Build history of the part. All positions in model axes, mm. Coordinates: 2 decimals unless noted, no trailing zeros. Write each loop counter-clockwise with the first axis right and the second up, starting at its lowest first coordinate (ties: lowest second). Pieces come first, ordered by that corner, then holes.
Autodesk Inventor part; units mm, degrees
ref_plane "YZ Plane" through (0, 0, 0) normal (1, 0, 0) x (0, 1, 0)
ref_plane "XZ Plane" through (0, 0, 0) normal (0, 1, 0) x (-1, 0, 0)
ref_plane "XY Plane" through (0, 0, 0) normal (0, 0, 1) x (1, 0, 0)
sketch "Sketch1" plane through (0, 0, 0) normal (1, 0, 0) x (0, 1, 0)
  circle A0 centre (0, 0) radius 57.15
  line L0 (5.3769, 1.4637) -> (3.9561, -3.9247)
  line L1 (3.9561, -3.9247) -> (-1.4208, -5.3884)
  line L2 (-1.4208, -5.3884) -> (-5.3769, -1.4637)
  line L3 (-5.3769, -1.4637) -> (-3.9561, 3.9247)
  line L4 (-3.9561, 3.9247) -> (1.4208, 5.3884)
  line L5 (1.4208, 5.3884) -> (5.3769, 1.4637)
  dimension "d0" = 114.3
  dimension "d1" = 9.652
extrude "Extrusion1" add sketch "Sketch1" along normal blind 6.35
sketch "Sketch2" plane through (6.35, 0, 0) normal (1, 0, 0) x (0, 0, -1)
  circle A0 centre (0, 0) radius 50.9905
  line L0 (3.9247, 3.9561) -> (5.3884, -1.4208)
  line L1 (5.3884, -1.4208) -> (1.4637, -5.3769)
  line L2 (1.4637, -5.3769) -> (-3.9247, -3.9561)
  line L3 (-3.9247, -3.9561) -> (-5.3884, 1.4208)
  line L4 (-5.3884, 1.4208) -> (-1.4637, 5.3769)
  line L5 (-1.4637, 5.3769) -> (3.9247, 3.9561)
  circle A1 centre (0, 0) radius 57.15
  dimension "d4" = 101.981
extrude "Extrusion2" add sketch "Sketch2" along normal blind 3.175 contours A0
sketch "Sketch3" plane through (0, 0, 0) normal (-1, 0, 0) x (0, 0, 1)
  circle A0 centre (0, 53.975) radius 1.397
  point P0 (0, 0)
  dimension "d7" = 2.794
  dimension "d8" = 53.975
extrude "Extrusion3" cut sketch "Sketch3" against normal blind 6.35
pattern_circular "Circular Pattern1" count 36 over 360 about axis through (-10, 0, 0) along (1, 0, 0) of "Extrusion3"
properties part number "wheel hub"
(1) Slice it at C-C, the plane z = -32. List the corners of the cut face in (x, y) (3 decimals).
(2) Slice it at A-A, the plane z = 0. Give the number of separate pieces and of enclosed holes in the cut face, and give its area (3 significant figures).
(3) Two-plate mould, pull along Z, no slides. Class faces 1 (the cylindrical face through (3.131, -52.51, -8.133)), 2 (the flat face through (0, -1, -12)): pulls with the +Z half, pulls with the -Z half, needs draft (parallel to the pull), parting line crosses it, or undercut.
(4) Probe L1, parallel to Y at x = 5.5, z = 10; L2, parallel to Y at x = 1.25, z = 9; L3, parallel to Z at x = 2.5, y = -46. List the from-to ranges inside material, lowest first.
(5) Flat gauge pins, fed straight in: P1, Ø2, axis at x = 5.5, y = -1.5, coming from the -Z side; P2, Ø3.5, axis at y = 9.37, z = 53.15, coming from the -X side; P3, Ø3.5, axis at y = 0, z = -53.975, coming from the +X side; P4, Ø1, axis at x = 5, y = 45.5, coming from the +Z side. Where does each tip first touch, or does it go through?
(6) Slice it at D-D, the plane y = 31.5. List the corners of the cut face in (x, z) (3 decimals), and give its area (3 significant figures).
Results:
1. outline: (0, -47.351) - (6.35, -47.351) - (6.35, -39.699) - (9.525, -39.699) - (9.525, 39.699) - (6.35, 39.699) - (6.35, 47.351) - (0, 47.351) - close
2. separate pieces: 4
2. enclosed holes: 0
2. area: 919 mm2
3. face 1: undercut
3. face 2: needs draft
4. L1: y = -56.27 to -54.4, -51.91 to 51.91, 54.4 to 56.27
4. L2: y = -56.44 to -54.5, -51.81 to 51.81, 54.5 to 56.44
4. L3: z = -33.91 to -28.17, -25.8 to 25.8, 28.17 to 33.91
5. P1: stops at z = -57.15
5. P2: stops at x = 0
5. P3: stops at x = 6.35
5. P4: stops at z = 35.23
6. outline: (0, -47.685) - (6.35, -47.685) - (6.35, -40.097) - (9.525, -40.097) - (9.525, 40.097) - (6.35, 40.097) - (6.35, 47.685) - (0, 47.685) - close
6. area: 860 mm2
